from build123d import *

# Parameters (mm, degrees)
F0_R     = 22.948461
F1_DEPTH = 50.8
F2_W     = 130.250856
F2_H     = 105.779626
F3_DEPTH = 25.4
F5_DEPTH = 127


with BuildPart() as f1:
    # F0 (on Top) → F1 (new body)
    with BuildSketch(Plane.XY):
        Circle(F0_R)
    extrude(amount=F1_DEPTH)

    # F2 (on Top) → F3 (join)
    with BuildSketch(Plane.XY):
        Rectangle(F2_W, F2_H)
    extrude(amount=F3_DEPTH)

    # F4 (on Front) → F5 (cut, symmetric)
    with BuildSketch(Plane.XZ):
        Polygon((31.802371, 53.156704), (-29.969381, 53.156704), (31.802371, 29.327836), (33.301385, 50.980239), (33.452064, 53.156704), align=None)
    extrude(amount=F5_DEPTH, both=True, mode=Mode.SUBTRACT)


solid = f1.part
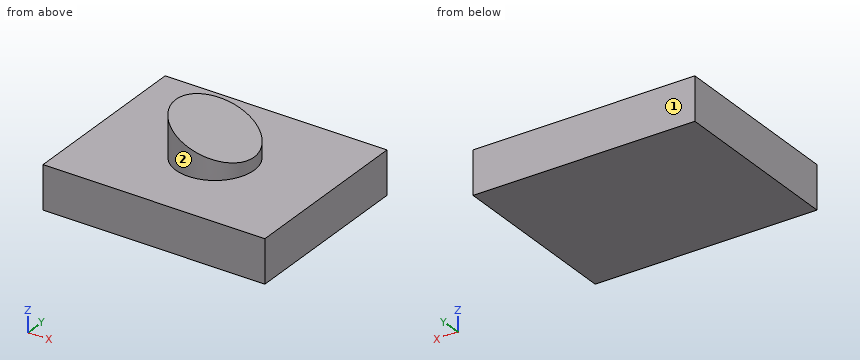
Work out the finished part from the listing and answer in its coordinate system (mm). Face numbers are marked on the shaded views. A direction names the side the tool comes from. Round coordinates to 2 decimals unless told otherwise and drop trailing zeros. Loops run counter-clockwise (first coordinate to the right, second up) from the corner with the lowest first, then second, coordinate; pieces in that order, holes last. Notation, with made-up numbers: M 78,-14.5 L 106,-14.5 A31 cw 106,12.5 Z; hole C 36.5,23 d10. An arc over 180 degrees is marked long. One line per question, with ' | ' between items. Start each with the question number.
(1) A cutting plane is placed at C-C on z = 30.5. Write down the section's boundary in (x, y), plus the area to 3 significant figures.
(2) A cutting plane is placed at D-D on y = 27. Write down the section's boundary in (x, z), plus the area to 3 significant figures.
(3) Flat-ended cylindrical pins translate along their axes: pin 1 Ø4 at (x, y) = (29.5, 34.5) entering from -Z; pin 2 Ø1.5 at (x, z) = (-12.5, 41) entering from -Y; pin 3 Ø12 at (y, z) = (-4.5, 33.5) entering from -X; pin 4 Ø12 at (x, y) = (34, -34) entering from +Z. Find the tip coordinate at first contact, or state that the pin passes through.
(4) A cutting plane is placed at A-A on y = 0. Write down the section's boundary in (x, z).
(5) A tool of negligible diameter and unlimited length cuts with its end or side. For the marked faces 1 and 2, from which of +Z, -Z, +X, -X, +Y, -Y can it reach the whole face along a straight path? Write none if from no direction.
(6) A cutting plane is placed at B-B on x = 14. Write down the section's boundary in (y, z).
(7) Find the intervals of material crossed by line 1 (Z direction, x = 36.5, y = -9.5); line 2 (Z direction, x = -21, y = 1); line 3 (Y direction, x = 12, z = 26.5), in increasing order.
Geometry check:
1) outline: C 0,0 d45.9 | area: 1,650 mm²
2) outline: M -65.13,0 L 65.13,0 L 65.13,25.4 L -65.13,25.4 Z | area: 3,310 mm²
3) pin 1: stops at z = 0 | pin 2: stops at y = -19.71 | pin 3: stops at x = -22.95 | pin 4: stops at z = 25.4
4) outline: M -65.13,0 L 65.13,0 L 65.13,25.4 L 22.95,25.4 L 22.95,32.74 L -22.95,50.45 L -22.95,25.4 L -65.13,25.4 Z
5) face 1: +Z, -Z, +X, -X, +Y | face 2: +Z
6) outline: M -52.89,0 L 52.89,0 L 52.89,25.4 L 18.18,25.4 L 18.18,36.2 L -18.18,36.2 L -18.18,25.4 L -52.89,25.4 Z
7) line 1: z = 0 to 25.4 | line 2: z = 0 to 49.7 | line 3: y = -19.56 to 19.56
